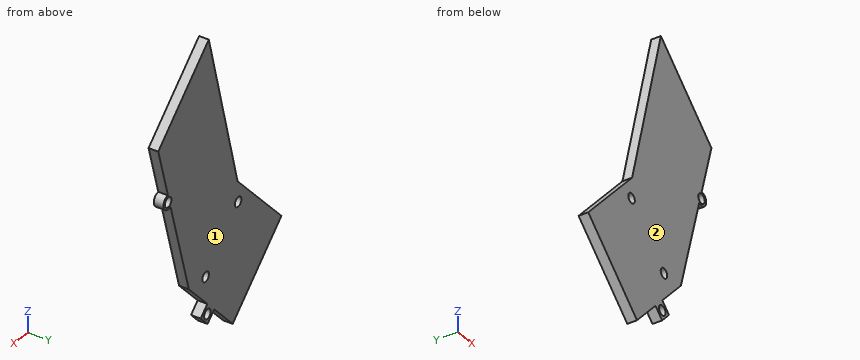
from build123d import *

# Parameters (mm, degrees)
SKETCH1_R           = 3.175
BOSS_EXTRUDE1_DEPTH = 6.35


with BuildPart() as part:
    # Sketch1 → Boss-Extrude1 (new body)
    with BuildSketch(Plane(origin=(0, 0, 0), x_dir=(1, 0, 0), z_dir=(0, 1, 0))):
        with BuildLine():
            Line((45.017746951, 2.631829887), (35.550660053, 36.209226482))
            ThreePointArc((35.550660053, 36.209226482), (39.762177432, 42.05307025), (33.11828595, 44.83625091))
            Line((33.11828595, 44.83625091), (15.243844224, 108.232438689))
            Line((15.243844224, 108.232438689), (-2.783728935, 127.479661752))
            Line((-2.783728935, 127.479661752), (3.678966496, 133.532831827))
            Line((3.678966496, 133.532831827), (-3.005742225, 140.669792455))
            Line((-3.005742225, 140.669792455), (-9.468437655, 134.61662238))
            Line((-9.468437655, 134.61662238), (-27.496010814, 153.863845442))
            Line((-27.496010814, 153.863845442), (-74.966911398, 109.401060841))
            Line((-74.966911398, 109.401060841), (-32.227053049, 63.769650553))
            Line((-32.227053049, 63.769650553), (-4.208751998, -43.475305064))
            Line((-4.208751998, -43.475305064), (45.017746951, 2.631829887))
        make_face()
        with Locations(Location((-2.894634056, 134.074815557, 0), (0, 0, 270))):
            Circle(SKETCH1_R, mode=Mode.SUBTRACT)
        with Locations(Location((35.334305242, 40.804639607, 0), (0, 0, 270))):
            Circle(SKETCH1_R, mode=Mode.SUBTRACT)
        with Locations(Location((-32.808552916, 77.429328599, 0), (0, 0, 270))):
            Circle(SKETCH1_R, mode=Mode.SUBTRACT)
        with Locations(Location((-1.199981142, 109.041759799, 0), (0, 0, 270))):
            Circle(SKETCH1_R, mode=Mode.SUBTRACT)
    extrude(amount=BOSS_EXTRUDE1_DEPTH)


solid = part.part
Design review of the part built by this model. Coordinates are the model's own, in mm. Face numbers are marked on the shaded views. Give positions to 0.01 mm unless a question says otherwise; leave off trailing zeros. Write each loop counter-clockwise with the first axis right and the second up, starting at its lowest first coordinate (ties: lowest second). Pieces come first, ordered by that corner, then holes. Notation, with made-up numbers: M 24,49 L 69,49 A27 cw 69,72 Z; hole C 14.5,-10.5 d8. An arc over 180 degrees is marked long. Answer as a JSON object with one key per item and string values. Group by question number.
1) We need section C-C (x = 29). Give the boundary of the cut face in (y, z).
2) We need section A-A (y = 1.75). Count the separate pieces of the cut face and the enclosed holes in it, and give its area (3 significant figures).
3) For line 1 along X through (y, z) = (4.5, -135); line 2 along Z through (x, y) = (-4, 2.75); line 3 along X through (y, z) = (4, -40), list the stretches that pass through material, from the lowest coordinate up.
4) We need section B-B (z = -54). Give the boundary of the cut face in (x, y).
5) Mouldability with a two-part tool opening along Y and no side actions: class the marked faces 1 and 2 as released by +Y, released by -Y, zero draft, split by the parting line, or undercut.
6) Clearance check with flat-ended pins moving along their axes: pin 1 Ø5 at (x, z) = (35.33, -40.8) entering from -Y; pin 2 Ø2 at (y, z) = (3.5, -128) entering from -X; pin 3 Ø1 at (y, z) = (3, 0) entering from -X; pin 4 Ø1 at (y, z) = (2, -81.5) entering from -X. State where each tip first meets the part, or that it passes through.
Answer key:
{
 "1": {"outline": "M 0,-59.44 L 6.35,-59.44 L 6.35,12.37 L 0,12.37 Z"},
 "2": {"separate pieces": "1", "enclosed holes": "4", "area": "10,500 mm²"},
 "3": {"line 1": "x = -47.64 to -9.83, -9.06 to -5.93, 0.14 to 2.3", "line 2": "z = -139.74 to -137.05, -131.1 to -110.54, -107.54 to 43.28", "line 3": "x = -26.02 to 32.26, 38.41 to 39.86"},
 "4": {"outline": "M -29.67,0 L 30.53,0 L 30.53,6.35 L -29.67,6.35 Z"},
 "5": {"face 1": "released by +Y", "face 2": "released by -Y"},
 "6": {"pin 1": "passes through", "pin 2": "stops at x = -56.18", "pin 3": "stops at x = -15.7", "pin 4": "stops at x = -49.3"}
}
